Autodesk Inventor part; units mm, degrees
ref_plane "YZ Plane" through (0, 0, 0) normal (1, 0, 0) x (0, 1, 0)
ref_plane "XZ Plane" through (0, 0, 0) normal (0, 1, 0) x (-1, 0, 0)
ref_plane "XY Plane" through (0, 0, 0) normal (0, 0, 1) x (1, 0, 0)
sketch "Esquisse1" plane through (0, 0, 0) normal (0, 0, 1) x (1, 0, 0)
  line L0 (0, 0) -> (0, 38.6276)
  line L1 (0, 38.6276) -> (16.5, 48.1538)
  line L2 (16.5, 48.1538) -> (13.5, 53.35)
  line L3 (13.5, 53.35) -> (-50.3694, 16.475)
  line L4 (-50.3694, 16.475) -> (-60.3694, 33.7955)
  line L5 (-60.3694, 33.7955) -> (-80.7, 22.0576)
  line L6 (-85.7, 13.3974) -> (-85.7, 0)
  line L7 (-85.7, 0) -> (0, 0)
  arc A0 (-80.7, 22.0576) -> (-85.7, 13.3974) centre (-75.7, 13.3974) ccw
  line L8 (-79.9, 0) -> (-39.75, 0) construction
  line L9 (-39.75, 0) -> (-39.75, 10.075) construction
  line L10 (-39.75, 10.075) -> (-79.9, 10.075) construction
  line L11 (-79.9, 10.075) -> (-79.9, 0) construction
  dimension "d0" = 20
  dimension "d1" = 73.75
  dimension "d3" = 6
  dimension "d4" = 16.5
  dimension "d7" = 85.7
  dimension "d32" = 40.15
  dimension "d33" = 5.8
  dimension "d34" = 10.075
  dimension "d35" = 6.4
  dimension "d38" = 120
  dimension "d39" = 10
extrude "Embase" add sketch "Esquisse1" along normal mid plane 40.2
mirror "Symétrie1" about plane through (-85.7, 0, 0) normal (0, -1, 0) of "Embase"
sketch "Esquisse2" plane through (0, 0, 20.1) normal (0, 0, 1) x (1, 0, 0)
  line L0 (-79.95, -10.075) -> (-39.8, -10.075)
  line L1 (-39.8, -10.075) -> (-39.8, 10.075)
  line L2 (-39.8, 10.075) -> (-79.95, 10.075)
  line L3 (-79.95, 10.075) -> (-79.95, -10.075)
  line L4 (0, 38.6276) -> (0, -38.6276)
  line L5 (-85.7, 13.3974) -> (-85.7, -13.3974)
  point P0 (0, 0)
  point P1 (-39.8, 0)
  point P2 (0, 0)
  dimension "d14" = 20.15
  dimension "d15" = 40.15
  dimension "d16" = 5.75
extrude "Passage profilé vertical" cut sketch "Esquisse2" against normal through all
sketch "Esquisse3" plane through (0, 0, 20.1) normal (0, 0, 1) x (1, 0, 0)
  line L0 (-31.8, -20.3371) -> (-31.8, 20.3371)
  line L1 (-31.8, 20.3371) -> (-3.9, 36.4452)
  line L2 (-3.9, 36.4452) -> (-3.9, -36.4452)
  line L3 (-31.8, -20.3371) -> (-3.9, -36.4452)
  line L4 (0, 38.6276) -> (0, -38.6276)
  line L5 (13.5, 53.35) -> (-50.3694, 16.475)
  line L6 (13.5, -53.35) -> (-50.3694, -16.475)
  point P0 (0, 0)
  dimension "d19" = 27.9
  dimension "d20" = 3.9
  dimension "d21" = 5.94
  dimension "d22" = 5.94
extrude "Passage courroie" cut sketch "Esquisse3" against normal through all
fillet "Congé1" radius 10 2 edges at (-31.8, -20.3371, 0) (-31.8, 20.3371, 0)
fillet "Congé1" radius 2 2 edges at (-3.9, -36.4452, 0) (-3.9, 36.4452, 0)
fillet "Congé1" radius 5 2 edges at (0, -38.6276, 0) (0, 38.6276, 0)
sketch "Esquisse7" plane through (0, 0, 20.1) normal (0, 0, 1) x (1, 0, 0)
  point P0 (0, 0)
  point P1 (-63, -20.5)
  point P2 (-63, 20.5)
  dimension "d51" = 20.5
  dimension "d52" = 63
  dimension "d53" = 20.5
  dimension "d54" = 63
hole "Passage axe" at (-63, -20.5, 20.1) at (-63, 20.5, 20.1) direction (0, 0, -1) diameter 12 end through all
sketch "Esquisse8" plane through (-85.7, 13.3974, -20.1) normal (-1, 0, 0) x (0, 0, 1)
  point P0 (20.1, -13.3974)
  point P1 (10.1, -13.3974)
  point P2 (30.1, -13.3974)
  dimension "d55" = 20
  dimension "d56" = 10
hole "Maintient profilé vertical" at (-85.7, 0, -10) at (-85.7, 0, 10) direction (1, 0, 0) diameter 5.5 end up to surface countersink diameter 9.5 countersink angle 90
sketch "Esquisse9" plane through (-50.3694, -16.475, -20.1) normal (-0.5, -0.8660254, 0) x (0.8660254, -0.5, 0)
  line L0 (0, 0) -> (73.75, 0)
  line L1 (73.75, 40.2) -> (0, 40.2)
  line L2 (73.75, 40.2) -> (73.75, 0)
  point P0 (35.3837, 20.1)
  point P1 (27.3, 30.1)
  point P2 (27.3, 10.3)
  point P3 (64.5, 30.1)
  point P4 (64.5, 10.3)
  dimension "d64" = 37.2
  dimension "d66" = 10.3
  dimension "d67" = 10.1
  dimension "d68" = 9.25
hole "Maintient profilé horizonal" at (-26.7269, -30.125, 10) at (-26.7269, -30.125, -9.8) at (5.4893, -48.725, 10) at (5.4893, -48.725, -9.8) direction (0.5, 0.8660254, 0) diameter 5.2 depth 8 tip angle 118
mirror "Symétrie2" about plane through (0, 0, 0) normal (0, 1, 0) of "Maintient profilé horizonal"
sketch "Esquisse10" plane through (0, -35.7408, 20.1) normal (1, 0, 0) x (0, 0, -1)
  line L0 (40.2, 71.4816) -> (40.2, 0)
  point P0 (20.1, 35.7408)
  point P1 (30.6, 35.7408)
  dimension "d76" = 9.6
hole "Perçage roulement a bille" at (0, 0, -10.5) direction (-1, 0, 0) diameter 10 depth 10 tip angle 118 counterbore diameter 11.5 counterbore depth 1
sketch "Esquisse11" plane through (0, -35.7408, 20.1) normal (1, 0, 0) x (0, 0, -1)
  circle A0 centre (30.6, 35.7408) radius 5 construction
  point P0 (20.1, 35.7408)
  point P1 (30.6, 25.7408)
  point P2 (30.6, 45.7408)
  dimension "d84" = 20
  dimension "d85" = 10
hole "Taraudage plaque de maintient" at (0, -10, -10.5) at (0, 10, -10.5) direction (-1, 0, 0) diameter 2.013 depth 7.6 tip angle 118
sketch "Esquisse12" plane through (-31.8, -14.5636, 20.1) normal (1, 0, 0) x (0, 0, -1)
  circle A0 centre (30.6, 14.5636) radius 5 construction
  point P0 (20.1, 14.5636)
hole "Perçage roulement a bille intérieur" at (-31.8, 0, -10.5) direction (-1, 0, 0) diameter 10.5 depth 3
equation "\"d22\" = d21"
properties part number "Coins superieur" material "Aluminium"
The model under review builds one solid part; all positions refer to its coordinate system, in mm. A direction names the side the tool comes from. Coordinates: 2 decimals unless noted, no trailing zeros. Loops run counter-clockwise (first coordinate to the right, second up) from the corner with the lowest first, then second, coordinate; pieces in that order, holes last. Notation, with made-up numbers: M -2,51 L 5,51 A14 ccw 5,58 Z; hole C -37.75,-21 d3. An arc over 180 degrees is marked long. Put each result on its own line as item: value. Start each with the question number.
Q1. For faces 1 (the cylindrical face through (-25.9, -27.13, -12.28)), 2 (the flat face through (-60, 10.075, 0)), 3 (the flat face through (-18.882, -34.654, -0.281)), 4 (the cylindrical face through (-2.47, -1.5, -15.27)), 5 (the cylindrical face through (0.688, 38.273, 0.281)), list the 3-axis set-ups (+Z, -Z, +X, -X, +Y, -Y) from which the entire face can be reached by the end or side of a thin tool; tool diameter is ignored.
Q2. Add section B-B (z = 1). Count the separate pieces of the cut face and the enclosed holes in it, and give its area (3 significant figures).
Q3. Wall thickness on line 1 (Z direction, x = -82.4, y = 0); line 2 (X direction, y = -8, z = -0.5); line 3 (Z direction, x = -2.45, y = 0): over which ranges is each line inside the solid? List them lowest first.
Q4. Add section D-D (y = 20.5). Write out the cut boundary in (x, z).
Q5. Add section C-C (x = -63). Write out the cut boundary in (y, z) (3 decimals), and give its area (3 significant figures).
Q6. The part is to be moulded in two halves that separate along Z. For faces 6 (the cylindrical face through (-81.8, 1.05, 12.54)), 7 (the flat face through (0, -1, 0)), say which applies: +Z half, -Z half, draft (parallel to the pull), parting line (faces both ways), or undercut.
Q7. Add section A-A (y = 7). Write out the cut boundary in (x, z).
Q8. Clearance check with flat-ended pins moving along their axes: pin 1 (3.5 mm diameter, centred on y = 0, z = 10, fed in from -X); pin 2 (2 mm diameter, centred on x = -20, z = -8.5, fed in from +Y); pin 3 (1 mm diameter, centred on y = 41, z = 15, fed in from +X). State where each tip first meets the part, or that it passes through.
Answers:
1. face 1: none
1. face 2: +Z, -Z
1. face 3: +Z, -Z, -Y
1. face 4: +X
1. face 5: +Z, -Z, +X
2. separate pieces: 1
2. enclosed holes: 4
2. area: 2,570 mm^2
3. line 1: z = -20.1 to -12.75, -7.25 to 7.25, 12.75 to 20.1
3. line 2: x = -85.7 to -79.95, -39.8 to -31.8, -3.9 to 0
3. line 3: z = -20.1 to -15.5, -5.5 to 20.1
4. outline: M -82.74,-20.1 L -69,-20.1 L -69,20.1 L -82.74,20.1 Z; M -57,-20.1 L -52.69,-20.1 L -52.69,20.1 L -57,20.1 Z; M -43.4,-20.1 L -29.85,-20.1 L -29.85,20.1 L -43.4,20.1 Z; M -3.9,-20.1 L 0,-20.1 L 0,20.1 L -3.9,20.1 Z
5. outline: M -32.277,-20.1 L -26.5,-20.1 L -26.5,20.1 L -32.277,20.1 Z; M -14.5,-20.1 L -10.075,-20.1 L -10.075,20.1 L -14.5,20.1 Z; M 10.075,-20.1 L 14.5,-20.1 L 14.5,20.1 L 10.075,20.1 Z; M 26.5,-20.1 L 32.277,-20.1 L 32.277,20.1 L 26.5,20.1 Z
5. area: 820 mm^2
6. face 6: undercut
6. face 7: draft
7. outline: M -85.7,-20.1 L -79.95,-20.1 L -79.95,20.1 L -85.7,20.1 Z; M -39.8,-20.1 L -31.8,-20.1 L -31.8,20.1 L -39.8,20.1 Z; M -3.9,-20.1 L 0,-20.1 L 0,20.1 L -3.9,20.1 Z
8. pin 1: stops at x = -39.8
8. pin 2: stops at y = 34.59
8. pin 3: stops at x = 4.98
